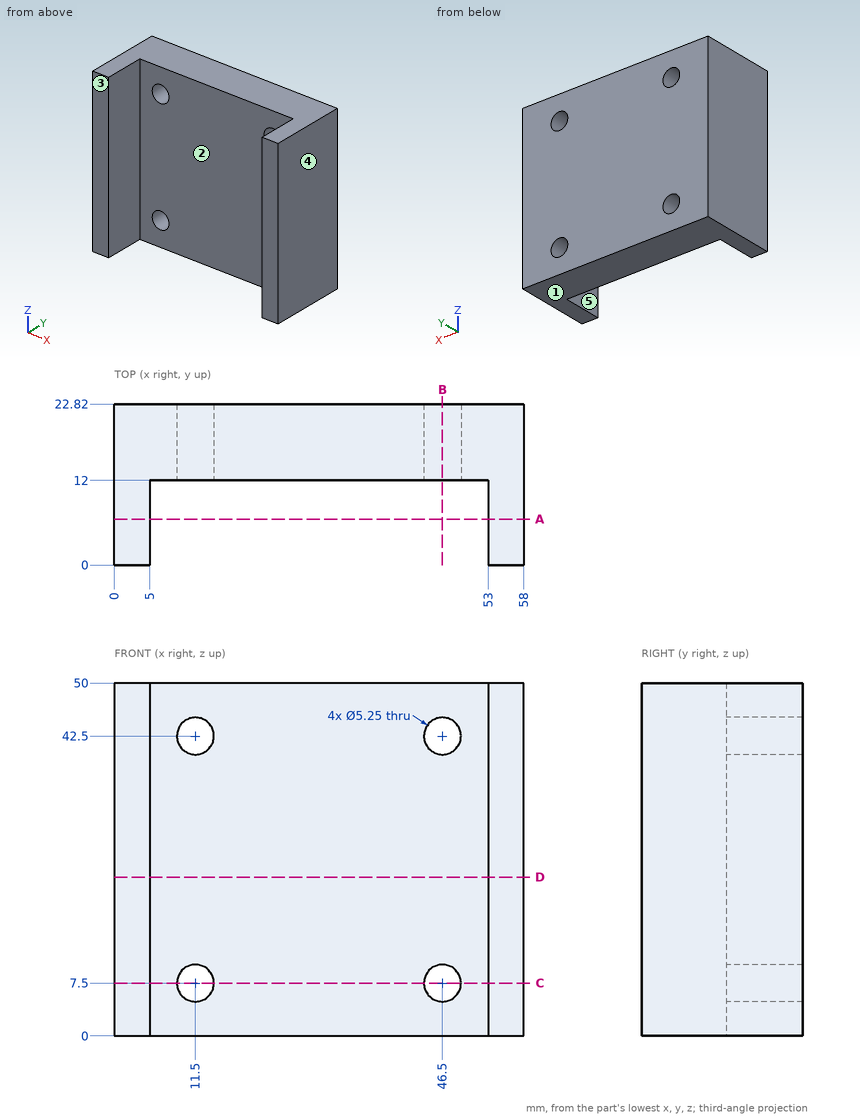
Geometry check sheet. Reference: drawing and pictorial views, mm from the part's lowest x, y, z. A direction names the side the tool comes from. Give positions to 0.01 mm unless a question says otherwise; leave off trailing zeros. Order: outer loops, then holes, each group sorted by start corner. A loop starts at its lowest first (then second) coordinate and runs counter-clockwise, first axis right, second up. Notation, with made-up numbers: M 19.25,0 L 58.25,0 A36 cw 58.25,36 Z; hole C 73.5,45 d4. An arc over 180 degrees is marked long. Use one line per item in the form item = value. Start each with the question number.
Q1. Access from +Z, -Z, +X, -X, +Y, -Y to the whole of each face (thin tool, end or side, straight path). Record for the marked faces 1 and 2.
Q2. Section check B-B (x = 46.5). Enter the section's corners in (y, z) (1 decimal).
Q3. Mould release check, pull along X, two halves, no side actions. Record for the marked faces 3, 4 and 5: +X half, -X half, draft (parallel to the pull), parting line (faces both ways), or undercut.
Q4. Section check D-D (z = 22.5). Enter the section's corners in (x, y).
Q5. Scan lines: line 1 along Z through (x, y) = (11.5, 15.75) (1 decimal); line 2 along X through (y, z) = (20.5, 42.5) (1 decimal); line 3 along X through (y, z) = (2.25, 22.5). Record each from-to range of solid material in increasing order. Write a range as [from, to].
Q6. Section check C-C (z = 7.5). Enter the section's corners in (x, y) (1 decimal).
Q7. Go/stop test with a flat-tipped pin: pin 1 Ø24 at (x, z) = (19.5, 17) entering from -Y. Record where the tip stops, or that it passes through.
Q8. Section check A-A (y = 6.5). Enter the section's corners in (x, z).
Evaluation:
q1.face_1 = -Z, +X, -X, +Y, -Y
q1.face_2 = +Z, -Z, -Y
q2.outline = M 12,0 L 22.8,0 L 22.8,4.9 L 12,4.9 Z; M 12,10.1 L 22.8,10.1 L 22.8,39.9 L 12,39.9 Z; M 12,45.1 L 22.8,45.1 L 22.8,50 L 12,50 Z
q3.face_3 = draft
q3.face_4 = +X half
q3.face_5 = undercut
q4.outline = M 0,0 L 5,0 L 5,12 L 53,12 L 53,0 L 58,0 L 58,22.82 L 0,22.82 Z
q5.line_1 = [0, 4.9], [10.1, 39.9], [45.1, 50]
q5.line_2 = [0, 8.9], [14.1, 43.9], [49.1, 58]
q5.line_3 = [0, 5], [53, 58]
q6.outline = M 0,0 L 5,0 L 5,12 L 8.9,12 L 8.9,22.8 L 0,22.8 Z; M 14.1,12 L 43.9,12 L 43.9,22.8 L 14.1,22.8 Z; M 49.1,12 L 53,12 L 53,0 L 58,0 L 58,22.8 L 49.1,22.8 Z
q7.pin_1 = 12
q8.outline = M 0,0 L 5,0 L 5,50 L 0,50 Z; M 53,0 L 58,0 L 58,50 L 53,50 Z
